```python
from build123d import *

# Parameters (mm, degrees)
SKETCH1_W           = 72.3
SKETCH1_H           = 72.3
BOSS_EXTRUDE1_DEPTH = 8.2
BOSS_EXTRUDE1_DRAFT = -8.77
SKETCH2_R           = 1.5
CUT_EXTRUDE1_DEPTH  = 10


with BuildPart() as part:
    # Sketch1 → Boss-Extrude1 (with draft: the straight prism first)
    with BuildSketch(Plane(origin=(0, 0, 0), x_dir=(1, 0, 0), z_dir=(0, 1, 0))):
        Rectangle(SKETCH1_W, SKETCH1_H)
    extrude(amount=BOSS_EXTRUDE1_DEPTH)
    # Boss-Extrude1: the draft: its side faces are tilted about the plane it starts from
    boss_extrude1_sides = [part.faces().sort_by_distance(p)[0] for p in [
        (-36.15, 4.1, 0),
        (0, 4.1, 36.15),
        (36.15, 4.1, 0),
        (0, 4.1, -36.15),
    ]]
    draft(boss_extrude1_sides, Plane(origin=(0, 0, 0), x_dir=(1, 0, 0), z_dir=(0, 1, 0)), BOSS_EXTRUDE1_DRAFT)

    # Sketch2 → Cut-Extrude1 (cut)
    with BuildSketch(Plane(origin=(0, 8.2, 0), x_dir=(1, 0, 0), z_dir=(0, 1, 0))):
        with Locations(Location((-33.066601018, 33.066601018, 0), (0, 0, 270))):
            Circle(SKETCH2_R)
        with Locations(Location((33.066601018, 33.066601018, 0), (0, 0, 270))):
            Circle(SKETCH2_R)
        with Locations(Location((33.066601018, -33.066601018, 0), (0, 0, 270))):
            Circle(SKETCH2_R)
        with Locations(Location((-33.066601018, -33.066601018, 0), (0, 0, 270))):
            Circle(SKETCH2_R)
    extrude(amount=-CUT_EXTRUDE1_DEPTH, mode=Mode.SUBTRACT)


solid = part.part
```
The model under review builds one solid part; all positions refer to its coordinate system, in mm. Round coordinates to 2 decimals unless told otherwise and drop trailing zeros. Loops run counter-clockwise (first coordinate to the right, second up) from the corner with the lowest first, then second, coordinate; pieces in that order, holes last. Notation, with made-up numbers: M 39,36.25 L 55,36.25 A25 cw 55,52.25 Z; hole C 25.5,23.5 d11. An arc over 180 degrees is marked long. Answer as a JSON object with one key per item and string values.
(1) Take a section at A-A on y = 3.5. Give the boundary of the cut face in (x, z).
Resolved:
{"outline": "M -36.69,-36.69 L 36.69,-36.69 L 36.69,36.69 L -36.69,36.69 Z; hole C -33.07,-33.07 d3; hole C -33.07,33.07 d3; hole C 33.07,-33.07 d3; hole C 33.07,33.07 d3"}
(2) Take a section at C-C on x = -26. Give the boundary of the cut face in (y, z), and give its area (3 significant figures).
Resolved:
{"outline": "M 0,-36.15 L 8.2,-37.42 L 8.2,37.42 L 0,36.15 Z", "area": "603 mm²"}
(3) To check wall thickness, follow line 1 along Z through (x, y) = (-16, 2.5); line 2 along Z through (x, y) = (-10, 1); line 3 along X through (y, z) = (7.25, -20.5). State the ranges of each line that lie inside material, in increasing order.
Resolved:
{"line 1": "-36.54 to 36.54", "line 2": "-36.3 to 36.3", "line 3": "-37.27 to 37.27"}
(4) Clearance check with flat-ended pins moving along their axes: P1, Ø2.5, axis at x = 33.07, z = 33.07, coming from the +Y side; P2, Ø4, axis at y = 1.5, z = 26, coming from the +X side; P3, Ø4, axis at x = 26, y = 3, coming from the -Z side; P4, Ø3, axis at x = -16.5, y = 3.5, coming from the +Z side. State where each tip first meets the part, or that it passes through.
Resolved:
{"P1": "through", "P2": "x = 36.69", "P3": "z = -36.92", "P4": "z = 36.92"}
(5) Take a section at B-B on z = -22.5. Give the boundary of the cut face in (x, y), and give its area (3 significant figures).
Resolved:
{"outline": "M -37.42,8.2 L -36.15,0 L 36.15,0 L 37.42,8.2 Z", "area": "603 mm²"}
